Build history of the part. All positions in model axes, mm. Round coordinates to 2 decimals unless told otherwise and drop trailing zeros. Write each loop counter-clockwise with the first axis right and the second up, starting at its lowest first coordinate (ties: lowest second). Pieces come first, ordered by that corner, then holes. Notation, with made-up numbers: (49.25, 26.5) - (84.25, 26.5) arc R20 cw to (84.25, 57.5) - close; hole circle Ø3 at (-20, -32.75). An arc over 180 degrees is marked (long way). One line per question, with ' | ' between items.
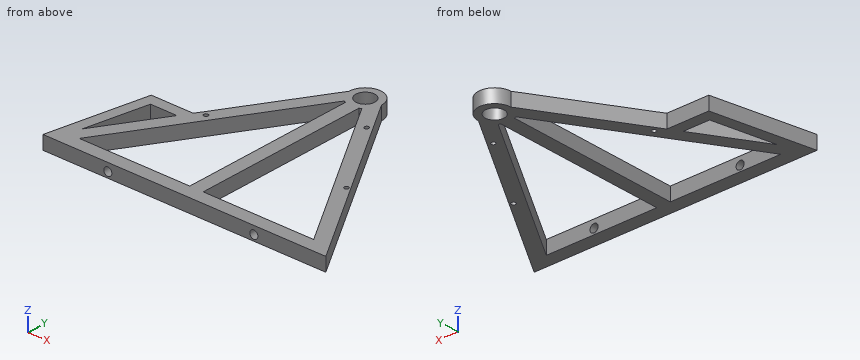
from build123d import *

# Parameters (mm, degrees)
F0_R     = 7
F1_DEPTH = 10
F3_D     = 6
F3_DEPTH = 12
F3_TIP   = 1.8025818571
F5_D     = 3.2
F5_DEPTH = 12
F5_TIP   = 0.9613769904


with BuildPart() as f1:
    # F0 (on Top) → F1 (new body)
    with BuildSketch(Plane.XY):
        with BuildLine():
            ThreePointArc((12, 0), (0, 12), (-12, 0))
            Line((-12, 0), (-59.3705538667, -76.4041191398))
            Line((-59.3705538667, -76.4041191398), (-90.5554051491, -76.4041191398))
            Line((-90.5554051491, -76.4041191398), (-105, -150))
            Line((-105, -150), (105, -150))
            Line((105, -150), (12, 0))
        make_face()
        Polygon((-93.0711311838, -130.7598890062), (-83.972927495, -84.4041191398), (-64.3305538667, -84.4041191398), align=None, mode=Mode.SUBTRACT)
        with BuildLine():
            Line((-87.0339471359, -140), (-6.4913960666, -10.0926595656))
            ThreePointArc((-6.4913960666, -10.0926595656), (-5.7601676478, -10.527130125), (-5, -10.9087121146))
            Line((-5, -10.9087121146), (-5, -140))
            Line((-5, -140), (-87.0339471359, -140))
        make_face(mode=Mode.SUBTRACT)
        with BuildLine():
            ThreePointArc((4.9999998882, -10.9087121659), (5.7601675939, -10.5271301545), (6.4913960666, -10.0926595656))
            Line((6.4913960666, -10.0926595656), (87.0339471359, -140))
            Line((87.0339471359, -140), (4.9999998882, -140))
            Line((4.9999998882, -140), (4.9999998882, -10.9087121659))
        make_face(mode=Mode.SUBTRACT)
        Circle(F0_R, mode=Mode.SUBTRACT)
    extrude(amount=F1_DEPTH)

    # F3
    with Locations(Plane.XZ.offset(150)):
        with Locations((-56.8714849651, 4.1602337733), (51.5690222383, 4.1602337733)):
            Hole(F3_D / 2, depth=F3_DEPTH)
            with Locations((0, 0, -(F3_DEPTH + F3_TIP / 2))):  # 118° drill point
                Cone(0, F3_D / 2, F3_TIP, mode=Mode.SUBTRACT)

    # F5
    with Locations(Plane(origin=(0, 0, 0), x_dir=(1, 0, 0), z_dir=(0, 0, -1))):
        with Locations((-52.6564307511, 73.3130574226), (23.0723669739, 24.6802578412), (60.8978777595, 83.5804338496)):
            Hole(F5_D / 2, depth=F5_DEPTH)
            with Locations((0, 0, -(F5_DEPTH + F5_TIP / 2))):  # 118° drill point
                Cone(0, F5_D / 2, F5_TIP, mode=Mode.SUBTRACT)


solid = f1.part
Q1. Drop flat-ended pins along their axis: pin 1 (5 mm diameter, centred on x = 48.5, z = 5.5, fed in from +Y); pin 2 (1.5 mm diameter, centred on y = -23.5, z = 6.5, fed in from +X) (3 decimals); pin 3 (5 mm diameter, centred on x = -78.5, z = 6.5, fed in from +Y); pin 4 (11 mm diameter, centred on x = 0, y = 0, fed in from +Z). Give the stop position or say it passes through.
Found:
pin 1: y = -54.84 | pin 2: x = 27.035 | pin 3: y = -76.4 | pin 4: through
Q2. Saw through at B-B, the plane x = -80.5. List the corners of the cut face in (y, z), then the cut area to 3 significant figures.
Found:
outline: (-150, 0) - (-140, 0) - (-140, 10) - (-150, 10) - close; (-129.46, 0) - (-110.48, 0) - (-110.48, 10) - (-129.46, 10) - close; (-84.4, 0) - (-76.4, 0) - (-76.4, 10) - (-84.4, 10) - close | area: 370 mm^2
Q3. Saw through at C-C, the plane y = -57. List the corners of the cut face in (x, z).
Found:
outline: (-47.34, 0) - (-35.57, 0) - (-35.57, 10) - (-47.34, 10) - close; (-5, 0) - (5, 0) - (5, 10) - (-5, 10) - close; (35.57, 0) - (47.34, 0) - (47.34, 10) - (35.57, 10) - close
Q4. Saw through at A-A, the plane x = 0. List the corners of the cut face in (y, z).
Found:
outline: (-150, 0) - (-7, 0) - (-7, 10) - (-150, 10) - close; (7, 0) - (12, 0) - (12, 10) - (7, 10) - close
Q5. Drill centre lines: L1, parallel to Y at x = -80, z = 9.5; L2, parallel to X at y = -35, z = 1.25; L3, parallel to X at y = -41.5, z = 6. Where is each one in solid material? Low to high. Write a range as from..to.
Found:
L1: -150..-140, -128.65..-109.68, -84.4..-76.4 | L2: -33.7..-21.93, -5..5, 21.93..33.7 | L3: -37.73..-25.96, -5..5, 25.96..37.73
